Geometry: final body of the model. Coordinates: model frame, mm. Face numbers are marked on the shaded views. A direction names the side the tool comes from. Give positions to 0.01 mm unless a question says otherwise; leave off trailing zeros. Order: outer loops, then holes, each group sorted by start corner. A loop starts at its lowest first (then second) coordinate and runs counter-clockwise, first axis right, second up. Notation, with made-up numbers: (-22.75, 55) -> (36.25, 55) arc R6 ccw to (36.25, 61) -> close; hole circle Ø5 at (-24, -8.5). An arc over 180 degrees is marked (long way). Answer in a Markdown table with one row per item. Add a question column.
Q1. Line query: line 1 along X through (y, z) = (22.9, 8); line 2 along Z through (x, y) = (-36.2, 23.65); line 3 along Z through (x, y) = (-48.5, 6.5). Output: solid intervals per line, ascending. Write a range as from..to.
Q2. Cut plane B-B on z = 9.5. Return the cut outline in (x, y) (1 decimal), and give its area (3 significant figures).
Q3. Cut plane A-A on x = -43.5. Return the cut outline in (y, z), and give its area (3 significant figures).
Q4. Pull-direction query (X, two-part tool) for the marked faces 1, 2 and 3; classes: +X half, -X half, draft (parallel to the pull), parting line (faces both ways), or undercut.
Q5. Cut plane D-D on z = 1. Return the cut outline in (x, y).
Q6. Cut plane C-C on x = -57. Return the cut outline in (y, z).
Q7. Contact query for flat-ended pins moving along their axis: P1, Ø5, axis at y = 26, z = 5.5, coming from the +X side; P2, Ø12, axis at x = -61.5, y = 7.5, coming from the -Z side; P3, Ø1.6, axis at x = -64.5, y = 23.5, coming from the +Z side; P4, Ø1.8, axis at y = 25.5, z = 7, coming from the -X side. Output: stop coordinate, or through.
Q8. Set-up query: the marked faces 4, 5, 6 and 7. Return all of +Z, -Z, +X, -X, +Y, -Y with unobstructed straight access to the full face (end or side cutting, diameter ignored); none if empty.
Autodesk Inventor part; units mm, degrees
ref_plane "YZ Plane" through (0, 0, 0) normal (1, 0, 0) x (0, 1, 0)
ref_plane "XZ Plane" through (0, 0, 0) normal (0, 1, 0) x (-1, 0, 0)
ref_plane "XY Plane" through (0, 0, 0) normal (0, 0, 1) x (1, 0, 0)
sketch "Boceto3" plane through (-69.7362, 30.866, 0) normal (0, 0, -1) x (-1, 0, 0)
  line L0 (-8.7362, 5.134) -> (-26.7362, 5.134)
  line L1 (-36.7362, -4.866) -> (-36.7362, -22.866)
  line L2 (-26.7362, -32.866) -> (-8.7362, -32.866)
  line L3 (1.2638, -22.866) -> (1.2638, -4.866)
  line L4 (1.2638, -23.3279) -> (1.2638, -4.4042) construction
  line L5 (-8.2744, 5.134) -> (-27.1981, 5.134) construction
  line L6 (-36.7362, -4.4042) -> (-36.7362, -23.3295)
  circle A0 centre (-8.7362, -22.866) radius 10.0001 construction
  arc A1 (-8.7362, -32.866) -> (1.2638, -22.866) centre (-8.7362, -22.866) ccw
  arc A2 (1.2638, -4.866) -> (-8.7362, 5.134) centre (-8.7362, -4.866) ccw
  arc A3 (-26.7362, 5.134) -> (-36.7362, -4.866) centre (-26.7362, -4.866) ccw
  arc A4 (-36.7362, -22.866) -> (-26.7362, -32.866) centre (-26.7362, -22.866) ccw
  point P0 (-69.7362, -30.866)
  point P1 (1.2638, 5.134)
  point P2 (-36.7362, 5.134)
  dimension "d3" = 10
  dimension "d4" = 10
extrude "Extrusión2" add sketch "Boceto3" against normal blind 2
sketch "Boceto5" plane through (-61, -2, 0) normal (0, -1, 0) x (1, 0, 0)
  line L0 (18, 0) -> (28, 0) construction
  line L1 (18.5, 0) -> (20.0893, 4.4576)
  line L2 (20.0893, 4.4576) -> (12.0357, 8.0433)
  line L3 (12.0357, 8.0433) -> (8.4546, 0)
  line L4 (18, 0) -> (0, 0) construction
  line L5 (8.4546, 0) -> (18.5, 0)
  point P0 (61, 0)
  dimension "d7" = 9.5
  dimension "d8" = 66
  dimension "d9" = 8.8157
  dimension "d16" = 70.378
  dimension "d17" = 10.0454
extrude "Extrusión3" add sketch "Boceto5" along normal blind 1 and the other way blind 2
sketch "Boceto6" plane through (-61, -3, 0) normal (0, -1, 0) x (1, 0, 0)
  circle A0 centre (16.8, 8) radius 2.8 construction
  circle A1 centre (16.8003, 7.9997) radius 4.8004
  point P0 (61, 0)
extrude "Extrusión4" add sketch "Boceto6" against normal blind 3
sketch "Boceto7" plane through (-61, -3, 0) normal (0, -1, 0) x (1, 0, 0)
  arc A0 (20.0563, 4.4723) -> (12, 7.9631) centre (16.8003, 7.9997) ccw
  point P0 (61, 0)
hole "Agujero1" at (-44.1997, -3, 7.9997) direction (0, 1, 0) diameter 5.5 end through all
sketch "Boceto8" plane through (-69.7362, 30.866, 2) normal (0, 0, 1) x (1, 0, 0)
  line L0 (36.5362, -8.866) -> (30.5362, -8.866)
  line L1 (30.5362, -8.866) -> (30.5362, -5.866)
  line L2 (30.5362, -5.866) -> (36.5362, -5.866)
  line L3 (36.5362, -5.866) -> (36.5362, -8.866)
  line L4 (36.7362, -22.866) -> (36.7362, -4.866) construction
  point P0 (69.7362, -30.866)
  dimension "d27" = 0.2
  dimension "d28" = 3
  dimension "d29" = 6
  dimension "d30" = 1
extrude "Extrusión5" add sketch "Boceto8" along normal blind 9
fillet "Empalme1" radius 2 2 edges at (-33.2, 23.5, 11) (-39.2, 23.5, 11)
sketch "Boceto9" plane through (-39.2, 22, 2) normal (0, -1, 0) x (1, 0, 0)
  line L0 (2, 9) -> (4, 9) construction
  line L1 (3, 9) -> (3, 0) construction
  line L2 (6, 0) -> (0, 0) construction
  point P0 (39.2, -2)
  point P1 (3, 6)
  dimension "d34" = 3
hole "Agujero2" at (-36.2, 22, 8) direction (0, 1, 0) diameter 2 end through all
sketch "Boceto10" plane through (-33.2, 22, 2) normal (1, 0, 0) x (0, 0, -1)
  line L0 (0, 3) -> (-7, 3) construction
  line L1 (-4, 3) -> (-1, 6)
  line L2 (-1, 6) -> (0, 6)
  line L3 (0, 6) -> (0, 3)
  line L4 (-4, 3) -> (0, 3)
  point P0 (2, -22)
  dimension "d42" = 45
  dimension "d43" = 1
  dimension "d44" = 3
extrude "Extrusión6" add sketch "Boceto10" against normal blind 6
pattern_linear "Patrón rectangular1" count 2 spacing 28.6 along (-1, 0, 0) of "Extrusión6", "Extrusión5", "Agujero2", "Empalme1"
properties part number "base"
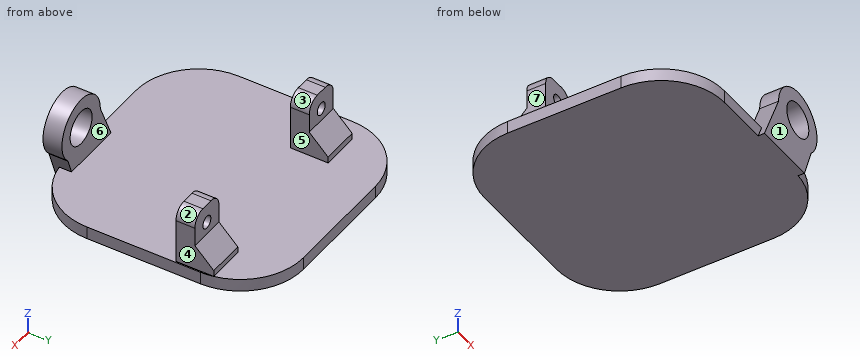
Completed:
| question | item | result |
|---|---|---|
| 1 | line 1 | x = -67.8..-65.8, -63.8..-61.8, -39.2..-37.2, -35.2..-33.2 |
| 1 | line 2 | z = 0..7, 9..11 |
| 1 | line 3 | z = 0..2 |
| 2 | outline | (-67.7, 22) -> (-61.9, 22) -> (-61.9, 25) -> (-67.7, 25) -> close; (-48.8, -3) -> (-46.5, -3) -> (-46.5, 0) -> (-48.8, 0) -> close; (-41.9, -3) -> (-39.6, -3) -> (-39.6, 0) -> (-41.9, 0) -> close; (-39.1, 22) -> (-33.3, 22) -> (-33.3, 25) -> (-39.1, 25) -> close |
| 2 | area | 48.8 mm² |
| 3 | outline | (-3, 0) -> (36, 0) -> (36, 2) -> (0, 2) -> (0, 5.34) -> (-3, 5.34) -> close; (-3, 10.66) -> (0, 10.66) -> (0, 12.75) -> (-3, 12.75) -> close |
| 3 | area | 94.3 mm² |
| 4 | face 1 | draft |
| 4 | face 2 | +X half |
| 4 | face 3 | undercut |
| 5 | outline | (-71, 8) arc R10 ccw to (-61, -2) -> (-52.1, -2) -> (-52.1, -3) -> (-42.14, -3) -> (-42.14, -1.96) arc R10 ccw to (-33, 8) -> (-33, 26) arc R10 ccw to (-43, 36) -> (-61, 36) arc R10 ccw to (-71, 26) -> close |
| 6 | outline | (-2, 0) -> (36, 0) -> (36, 2) -> (-2, 2) -> close |
| 7 | P1 | stops at x = -33.2 |
| 7 | P2 | stops at z = 0 |
| 7 | P3 | stops at z = 11 |
| 7 | P4 | stops at x = -67.8 |
| 8 | face 4 | +Z, +X, +Y, -Y |
| 8 | face 5 | +Z, +Y, -Y |
| 8 | face 6 | +Z, +X, -X, +Y |
| 8 | face 7 | +Z, -X, +Y, -Y |
